```python
from build123d import *
from build123d.topology import SkipClean

# Parameters (mm, degrees)
SKETCH1_R           = 50
BOSS_EXTRUDE1_DEPTH = 7
BOSS_EXTRUDE2_START = 12.6
SKETCH2_R           = 2.5
BOSS_EXTRUDE2_DEPTH = 12.6
CIRPATTERN1_COUNT   = 12
SKETCH3_R           = 12
CUT_EXTRUDE1_DEPTH  = 72.824508352
SKETCH4_R           = 31.5
SKETCH4_R_2         = 16.5
CUT_EXTRUDE2_DEPTH  = 3
BOSS_EXTRUDE3_START = -4.2
SKETCH5_R           = 12
SKETCH5_R_2         = 8.5
BOSS_EXTRUDE3_DEPTH = 2.8
SCALE1_SCALE        = 0.4


with BuildPart() as part:
    # Sketch1 → Boss-Extrude1 (new body)
    with BuildSketch(Plane.XY):
        Circle(SKETCH1_R)
    extrude(amount=-BOSS_EXTRUDE1_DEPTH)

    # Sketch2 → Boss-Extrude2 (add)
    with BuildSketch(Plane.XY.offset(BOSS_EXTRUDE2_START)):
        with BuildLine():
            Line((44.72775, 4.942507454), (48.490092946, 5.358254011))
            ThreePointArc((48.490092946, 5.358254011), (49.383550497, 5.092810123), (49.817513468, 4.267944684))
            ThreePointArc((49.817513468, 4.267944684), (50, 0), (49.817513468, -4.267944684))
            ThreePointArc((49.817513468, -4.267944684), (49.383550497, -5.092810123), (48.490092946, -5.358254011))
            Line((48.490092946, -5.358254011), (44.72775, -4.942507454))
            ThreePointArc((44.72775, -4.942507454), (40.05, 0), (44.72775, 4.942507454))
        make_face()
        with Locations((45, 0)):
            Circle(SKETCH2_R, mode=Mode.SUBTRACT)
    boss_extrude2 = extrude(amount=-BOSS_EXTRUDE2_DEPTH)

    # CirPattern1: Boss-Extrude2 ×12 about axis
    with SkipClean():  # the faces are left unmerged after this step: merging them gives an invalid solid
        cirpattern1_axis = Axis((0, 0, 0), (0, 0, 1))
        for i in range(1, CIRPATTERN1_COUNT):
            add(boss_extrude2.rotate(cirpattern1_axis, i * 360 / CIRPATTERN1_COUNT))

    # Sketch3 → Cut-Extrude1 (cut, through all)
    with SkipClean():  # the faces are left unmerged after this step: merging them gives an invalid solid
        with BuildSketch(Plane.XY):
            Circle(SKETCH3_R)
        extrude(amount=-CUT_EXTRUDE1_DEPTH, mode=Mode.SUBTRACT)

    # Sketch4 → Cut-Extrude2 (cut)
    with SkipClean():  # the faces are left unmerged after this step: merging them gives an invalid solid
        with BuildSketch(Plane.XY):
            Circle(SKETCH4_R)
            Circle(SKETCH4_R_2, mode=Mode.SUBTRACT)
        extrude(amount=-CUT_EXTRUDE2_DEPTH, mode=Mode.SUBTRACT)

    # Sketch5 → Boss-Extrude3 (add)
    with SkipClean():  # the faces are left unmerged after this step: merging them gives an invalid solid
        with BuildSketch(Plane.XY.offset(BOSS_EXTRUDE3_START)):
            Circle(SKETCH5_R)
            Circle(SKETCH5_R_2, mode=Mode.SUBTRACT)
        extrude(amount=-BOSS_EXTRUDE3_DEPTH)


with BuildPart() as part_1:
    # Scale1: scaled about (0, 0, -1.929689798)
    add(part.part.scale(SCALE1_SCALE).moved(Location((0, 0, -1.157813879))))


solid = part_1.part
```
Could you check a few things on this model? Use its own coordinates, in mm. A direction names the side the tool comes from. Round coordinates to 2 decimals unless told otherwise and drop trailing zeros. Loops run counter-clockwise (first coordinate to the right, second up) from the corner with the lowest first, then second, coordinate; pieces in that order, holes last. Notation, with made-up numbers: (-13.75, 5) - (2.25, 5) arc R26 ccw to (2.25, 25) - close; hole circle Ø9 at (0, 51). An arc over 180 degrees is marked (long way). Answer in a Markdown table with one row per item. Add a question column.
(1) I'm going to push flat-ended pins straight in: pin 1 (4 mm diameter, centred on x = 2.5, z = 0.5, fed in from +Y); pin 2 (1.6 mm diameter, centred on x = -18, y = 0, fed in from +Z); pin 3 (3 mm diameter, centred on x = -6.5, z = 0, fed in from -Y). Where does each tip first touch, or does it pass through?
(2) If we section it at B-B (z = 1.75): State how many separate pieces and enclosed holes the cut face has, plus the area to 3 significant figures.
(3) If we section it at C-C (x = 9): Please give me the cut outline in (y, z), plus the area to 3 significant figures.
(4) I need wall thicknesses on line 1 along Y through (x, z) = (9, 2.4); line 2 along Y through (x, z) = (0, -1.7); line 3 along X through (y, z) = (15, 3.5). Which ranges of each line are inside material? Lowest first, please.
(5) If we mould it in two halves opening along Y, with no side actions, what happens to faces 4 (the face through (-9, -17, 3.882)), 5 (the face through (7.542, -17.186, 1.397)), 6 (the face through (16.58, 9.13, 1.4))? For each: pulls with the +Y half, pulls with the -Y half, needs draft (parallel to the pull), parting line crosses it, or undercut.
(6) For faces 1 (the face through (4, 0, -3.958)), 2 (the face through (-16.58, -9.13, 1.4)), 3 (the face through (11.1, -15.11, 1.4)), which set-ups out of +Z, -Z, +X, -X, +Y, -Y let a thin tool reach every point of the face, with its end or its side?
Model answer:
| question | item | result |
|---|---|---|
| 1 | pin 1 | stops at y = 19.99 |
| 1 | pin 2 | stops at z = -1.16 |
| 1 | pin 3 | stops at y = -19.22 |
| 2 | separate pieces | 12 |
| 2 | enclosed holes | 12 |
| 2 | area | 134 mm² |
| 3 | outline | (-17.86, -3.96) - (17.86, -3.96) - (17.86, 3.88) - (16.59, 3.88) - (16.59, -1.16) - (14.59, -1.16) - (14.59, 3.88) - (13.61, 3.88) - (13.61, -1.16) - (8.82, -1.16) - (8.82, -2.36) - (-8.82, -2.36) - (-8.82, -1.16) - (-13.61, -1.16) - (-13.61, 3.88) - (-14.59, 3.88) - (-14.59, -1.16) - (-16.59, -1.16) - (-16.59, 3.88) - (-17.86, 3.88) - close |
| 3 | area | 102 mm² |
| 4 | line 1 | y = -17.86 to -16.59, -14.59 to -13.61, 13.61 to 14.59, 16.59 to 17.86 |
| 4 | line 2 | y = -20 to -12.6, -6.6 to -4.8, 4.8 to 6.6, 12.6 to 20 |
| 4 | line 3 | x = -11.02 to -9.81, -8.19 to -7.11, 7.11 to 8.19, 9.81 to 11.02 |
| 5 | face 4 | needs draft |
| 5 | face 5 | pulls with the -Y half |
| 5 | face 6 | undercut |
| 6 | face 1 | -Z, +X, -X, +Y, -Y |
| 6 | face 2 | +Z |
| 6 | face 3 | +Z, +X |
